```python
from build123d import *

# Parameters (mm, degrees)
SKETCH4_W           = 30
SKETCH4_H           = 30
BOSS_EXTRUDE2_DEPTH = 20
SKETCH5_R           = 14
CUT_EXTRUDE1_DEPTH  = 47.904157598
SKETCH6_W           = 2
SKETCH6_H           = 1
BOSS_EXTRUDE3_DEPTH = 1
SHELL6_START        = 2
SHELL6_DEPTH        = 26
FILLET1_R           = 0.5
CUT_EXTRUDE2_DEPTH  = 4
CUT_EXTRUDE11_START = -2
CUT_EXTRUDE11_DEPTH = 2
BOSS_EXTRUDE4_DEPTH = 3
SKETCH12_W          = 1.5
SKETCH12_H          = 1.5


# Read off the part's stored shape, not the designer's step: Shell6
with BuildPart() as part:
    # Sketch4 → Boss-Extrude2 (new body)
    with BuildSketch(Plane.XY):
        with Locations((15, 15)):
            Rectangle(SKETCH4_W, SKETCH4_H)
    extrude(amount=-BOSS_EXTRUDE2_DEPTH)

    # Sketch5 → Cut-Extrude1 (cut, through all)
    with BuildSketch(Plane(origin=(30, 0, 0), x_dir=(0, 0, -1), z_dir=(1, 0, 0))):
        with Locations((20, 15)):
            Circle(SKETCH5_R)
    extrude(amount=-CUT_EXTRUDE1_DEPTH, mode=Mode.SUBTRACT)

    # Sketch6 → Boss-Extrude3 (add)
    with BuildSketch(Plane.XY):
        with Locations((23.5, 15)):
            Rectangle(SKETCH6_W, SKETCH6_H)
        with Locations((6.5, 15)):
            Rectangle(SKETCH6_W, SKETCH6_H)
    extrude(amount=BOSS_EXTRUDE3_DEPTH)

    # Shell6 outline → Shell6 (cut)
    with BuildSketch(Plane.YZ.offset(SHELL6_START)):
        with BuildLine():
            Line((28, -2), (2, -2))
            Line((2, -2), (2, -10.672620947))
            ThreePointArc((2, -10.672620947), (15, -4), (28, -10.672620947))
            Line((28, -10.672620947), (28, -2))
        make_face()
    extrude(amount=SHELL6_DEPTH, mode=Mode.SUBTRACT)

    # Fillet1
    fillet1_edges = [part.edges().sort_by_distance(p)[0] for p in [
        (23.5, 15.5, 1),
        (23.5, 14.5, 1),
        (6.5, 15.5, 1),
        (6.5, 14.5, 1),
    ]]
    fillet(fillet1_edges, radius=FILLET1_R - 0.0001)  # a hair under: the kernel refuses the full size

    # Sketch7 → Revolve1 (revolve)
    with BuildSketch(Plane(origin=(0, 15, 0), x_dir=(-1, 0, 0), z_dir=(0, -1, 0))):
        Polygon((0, 0), (0, -4), (-5, -4), (-5, -2), (-3, -2), (-3, 0), align=None)
    revolve(axis=Axis((15, 15, 0), (0, 0, 1)))

    # Sketch9 → Cut-Extrude2 (cut)
    with BuildSketch(Plane.XY.offset(4)):
        with BuildLine():
            Line((6.396353455, 27.287280664), (9.264235636, 23.191520443))
            ThreePointArc((9.264235636, 23.191520443), (15, 25), (20.735764364, 23.191520443))
            Line((20.735764364, 23.191520443), (23.603646545, 27.287280664))
            ThreePointArc((23.603646545, 27.287280664), (15, 30), (6.396353455, 27.287280664))
        make_face()
    cut_extrude2 = extrude(amount=-CUT_EXTRUDE2_DEPTH, mode=Mode.SUBTRACT)

    # Mirror1: Cut-Extrude2 across plane
    add(cut_extrude2.mirror(Plane(origin=(0, 15, 0), x_dir=(0, 0, 1), z_dir=(0, -1, 0))), mode=Mode.SUBTRACT)

    # Sketch10 → Cut-Extrude11 (cut)
    with BuildSketch(Plane.XY.offset(CUT_EXTRUDE11_START)):
        with BuildLine():
            Line((11, 19), (3.686291501, 19))
            ThreePointArc((3.686291501, 19), (3, 15), (3.686291501, 11))
            Line((3.686291501, 11), (11, 11))
            Line((11, 11), (11, 11.5))
            Line((11, 11.5), (4.04554885, 11.5))
            ThreePointArc((4.04554885, 11.5), (3.5, 15), (4.04554885, 18.5))
            Line((4.04554885, 18.5), (11, 18.5))
            Line((11, 18.5), (11, 19))
        make_face()
        with BuildLine():
            Line((26.313708499, 19), (19, 19))
            Line((19, 19), (19, 18.5))
            Line((19, 18.5), (25.95445115, 18.5))
            ThreePointArc((25.95445115, 18.5), (26.5, 15), (25.95445115, 11.5))
            Line((25.95445115, 11.5), (19, 11.5))
            Line((19, 11.5), (19, 11))
            Line((19, 11), (26.313708499, 11))
            ThreePointArc((26.313708499, 11), (27, 15), (26.313708499, 19))
        make_face()
    extrude(amount=CUT_EXTRUDE11_DEPTH, mode=Mode.SUBTRACT)

    # Sketch11 → Boss-Extrude4 (add)
    with BuildSketch(Plane(origin=(0, 30, 0), x_dir=(1, 0, 0), z_dir=(0, 1, 0))):
        with BuildLine():
            Line((25, 20), (5, 20))
            ThreePointArc((5, 20), (15, 10), (25, 20))
        make_face()
    boss_extrude4 = extrude(amount=BOSS_EXTRUDE4_DEPTH)

    # Sketch12 → Cut-Revolve1 (revolve, cut)
    with BuildSketch(Plane(origin=(0, 0, -20), x_dir=(-1, 0, 0), z_dir=(0, 0, -1))):
        with Locations((-5.75, 30.75)):
            Rectangle(SKETCH12_W, SKETCH12_H)
    cut_revolve1 = revolve(axis=Axis((15, 33, -20), (0, -1, 0)), mode=Mode.SUBTRACT)

    # Mirror2: Boss-Extrude4, Cut-Revolve1 across plane
    add(boss_extrude4.mirror(Plane(origin=(0, 15, 0), x_dir=(0, 0, 1), z_dir=(0, -1, 0))))
    add(cut_revolve1.mirror(Plane(origin=(0, 15, 0), x_dir=(0, 0, 1), z_dir=(0, -1, 0))), mode=Mode.SUBTRACT)


solid = part.part
```
Source: CAD feature listing. Evaluate the final solid. Frame: model axes, mm. A direction names the side the tool comes from. Round coordinates to 2 decimals unless told otherwise and drop trailing zeros. Loops run counter-clockwise (first coordinate to the right, second up) from the corner with the lowest first, then second, coordinate; pieces in that order, holes last.
1. Section query B-B on x = 15. Output: boundary loops of the cut face in (y, z).
2. Section query A-A on z = -3. Output: boundary loops of the cut face in (x, y).
3. Mould query, pull axis Z, two halves, no side actions, for faces 1 (the flat face through (23, 11, -1)), 2 (the cylindrical face through (15, 32, -10)), 3 (the flat face through (22.47, 25.67, 2.47)). Classes: released by +Z, released by -Z, zero draft, split by the parting line, or undercut.
4. Contact query for flat-ended pins moving along their axis: pin 1 (1.6 mm diameter, centred on x = 9, z = -1, fed in from +Y); pin 2 (7 mm diameter, centred on x = 10.5, z = -8, fed in from -Y); pin 3 (0.6 mm diameter, centred on x = 23, z = 0, fed in from -Y); pin 4 (5 mm diameter, centred on x = 5.5, y = 19, fed in from -Z). Output: stop coordinate, or through.
5. Ray query, L1, parallel to Z at x = 10.25, y = 14.5; L2, parallel to Y at x = 4.25, z = -9.25; L3, parallel to Y at x = 22, z = -3.25. Return the intervals inside material, ascending.
6. Access query for faces 4 (the flat face through (22.47, 4.33, 2.47)), 5 (the cylindrical face through (30, 15, 2)), 6 (the cylindrical face through (15.187, -0.76, -11.502)), 7 (the flat face through (7.492, 25.723, 2.472)), 8 (the cylindrical face through (15, 15, -4)). Directions: +Z, -Z, +X, -X, +Y, -Y. A direction counts if a zero-diameter tool reaches every point of the face in a straight line with its end or side. Return the directions, or none.
7. Section query C-C on x = 4.5. Output: boundary loops of the cut face in (y, z).
8. Section query D-D on z = -15. Output: boundary loops of the cut face in (x, y).
Answers below:
1. outline: (-3, -20) - (1, -20) arc R14 cw to (29, -20) - (33, -20) - (33, -10) - (31.5, -10) - (31.5, -11.5) - (30, -11.5) - (30, 0) - (0, 0) - (0, -11.5) - (-1.5, -11.5) - (-1.5, -10) - (-3, -10) - close; hole (2, -10.67) arc R16 cw to (28, -10.67) - (28, -2) - (2, -2) - close
2. outline: (0, 0) - (30, 0) - (30, 30) - (0, 30) - close; hole (2, 2) - (28, 2) - (28, 28) - (2, 28) - close
3. face 1: undercut
3. face 2: released by +Z
3. face 3: zero draft
4. pin 1: stops at y = 30
4. pin 2: stops at y = -3
4. pin 3: stops at y = 0
4. pin 4: stops at z = -7.6
5. L1: z = -6.01 to -4.01, -2 to 0
5. L2: y = 0 to 2, 3.15 to 6.03, 23.97 to 26.85, 28 to 30
5. L3: y = 0 to 2, 28 to 30
6. face 4: +Z, -Y
6. face 5: +Z, +X
6. face 6: +Z
6. face 7: +Z, +Y
6. face 8: none
7. outline: (0, -20) - (1, -20) arc R14 cw to (29, -20) - (30, -20) - (30, 0) - (25.71, 0) - (25.71, 4) - (4.29, 4) - (4.29, 0) - (0, 0) - close; (11.5, -2) - (18.5, -2) - (18.5, 0) - (11.5, 0) - close; hole (2, -10.67) arc R16 cw to (28, -10.67) - (28, -2) - (19, -2) - (19, 0) - (20.81, 0) - (20.81, 2) - (9.19, 2) - (9.19, 0) - (11, 0) - (11, -2) - (2, -2) - close
8. outline: (0, 0) - (8.13, 0) - (8.13, -1.5) - (6.34, -1.5) - (6.34, -3) - (23.66, -3) - (23.66, -1.5) - (21.87, -1.5) - (21.87, 0) - (30, 0) - (30, 1.92) - (0, 1.92) - close; (0, 28.08) - (30, 28.08) - (30, 30) - (21.87, 30) - (21.87, 31.5) - (23.66, 31.5) - (23.66, 33) - (6.34, 33) - (6.34, 31.5) - (8.13, 31.5) - (8.13, 30) - (0, 30) - close
